```python
from build123d import *

# Parameters (mm, degrees)
SKETCH_1_W          = 45
SKETCH_1_H          = 40
EXTRUDE_1_DEPTH     = 20
SKETCH_2_W          = 45
SKETCH_2_H          = 10
CUT_EXTRUDE_1_DEPTH = 32
SKETCH_3_W          = 45
SKETCH_3_H          = 5
EXTRUDE_2_DEPTH     = 5
SKETCH_4_R          = 1.5
CUT_EXTRUDE_2_DEPTH = 44.934610502
CHAMFER_1_SIZE      = 10


with BuildPart() as part:
    # 草图1 → 凸台-拉伸1 (new body)
    with BuildSketch(Plane(origin=(0, 0, 0), x_dir=(1, 0, 0), z_dir=(0, 1, 0))):
        Rectangle(SKETCH_1_W, SKETCH_1_H)
    extrude(amount=EXTRUDE_1_DEPTH)

    # 草图2 → 切除-拉伸1 (cut)
    with BuildSketch(Plane(origin=(0, 0, -20), x_dir=(-1, 0, 0), z_dir=(0, 0, -1))):
        with Locations((0, 15)):
            Rectangle(SKETCH_2_W, SKETCH_2_H)
    extrude(amount=-CUT_EXTRUDE_1_DEPTH, mode=Mode.SUBTRACT)

    # 草图3 → 凸台-拉伸2 (add)
    with BuildSketch(Plane(origin=(0, 10, 0), x_dir=(1, 0, 0), z_dir=(0, 1, 0))):
        with Locations((0, 17.5)):
            Rectangle(SKETCH_3_W, SKETCH_3_H)
    extrude(amount=EXTRUDE_2_DEPTH)

    # 草图4 → 切除-拉伸2 (cut, through all)
    with BuildSketch(Plane(origin=(0, 0, 12), x_dir=(-1, 0, 0), z_dir=(0, 0, -1))):
        with Locations((0, 15)):
            Circle(SKETCH_4_R)
    extrude(amount=-CUT_EXTRUDE_2_DEPTH, mode=Mode.SUBTRACT)

    # 倒角1
    chamfer_1_edges = [part.edges().sort_by_distance(p)[0] for p in [
        (-22.5, 10, 20),
    ]]
    chamfer(chamfer_1_edges, length=CHAMFER_1_SIZE)


solid = part.part
```
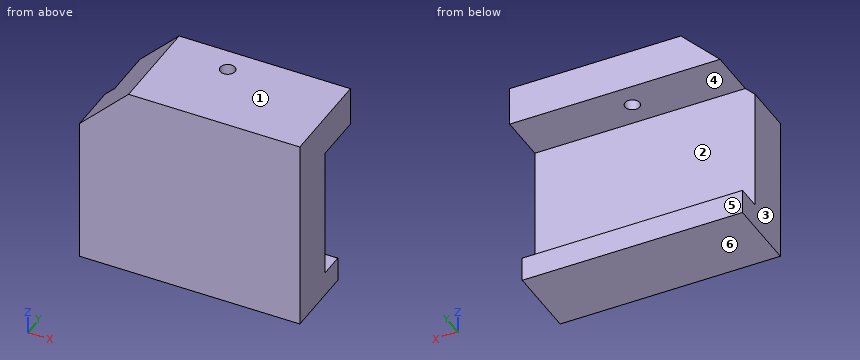
The model under review builds one solid part; all positions refer to its coordinate system, in mm. Face numbers are marked on the shaded views. A direction names the side the tool comes from. Give positions to 0.01 mm unless a question says otherwise; leave off trailing zeros. Loops run counter-clockwise (first coordinate to the right, second up) from the corner with the lowest first, then second, coordinate; pieces in that order, holes last. Notation, with made-up numbers: (11.25, 18) - (50.25, 18) arc R12 ccw to (50.25, 27) - close; hole circle Ø11 at (-5, 68.25). An arc over 180 degrees is marked (long way). Answer as a JSON object with one key per item and string values.
Q1. Add section A-A on x = 0. State the section outline as (y, z) points, plus the area to 3 significant figures.
Worked out:
{"outline": "(0, -20) - (15, -20) - (15, -15) - (10, -15) - (10, 12) - (13.5, 12) - (13.5, 20) - (0, 20) - close; (16.5, 12) - (20, 12) - (20, 20) - (16.5, 20) - close", "area": "481 mm^2"}
Q2. Mouldability with a two-part tool opening along Z and no side actions: class the marked faces 1, 2, 3 and 4 as +Z half, -Z half, draft (parallel to the pull), parting line (faces both ways), or undercut.
Worked out:
{"face 1": "+Z half", "face 2": "undercut", "face 3": "draft", "face 4": "undercut"}
Q3. Add section D-D on x = -8. State the section outline as (y, z) points.
Worked out:
{"outline": "(0, -20) - (15, -20) - (15, -15) - (10, -15) - (10, 12) - (20, 12) - (20, 20) - (0, 20) - close"}
Q4. To check wall thickness, follow line 1 along Y through (x, z) = (0, 16); line 2 along Z through (x, y) = (-10.5, 14); line 3 along Y through (x, z) = (7.5, 7.5). State the ranges of each line that lie inside material, in increasing order.
Worked out:
{"line 1": "y = 0 to 13.5, 16.5 to 20", "line 2": "z = -20 to -15, 12 to 20", "line 3": "y = 0 to 10"}
Q5. For the marked faces 5 and 6, list the 3-axis set-ups (+Z, -Z, +X, -X, +Y, -Y) from which the entire face can be reached by the end or side of a thin tool; tool diameter is ignored.
Worked out:
{"face 5": "-Z, +X, -X, +Y", "face 6": "-Z, +X, -X, +Y, -Y"}
Q6. Add section C-C on y = 11.75. State the section outline as (x, z) points.
Worked out:
{"outline": "(-22.5, -20) - (22.5, -20) - (22.5, -15) - (-22.5, -15) - close; (-20.5, 12) - (22.5, 12) - (22.5, 20) - (-12.5, 20) - close"}
Q7. Add section B-B on z = 14. State the section outline as (x, y) points.
Worked out:
{"outline": "(-18.5, 0) - (22.5, 0) - (22.5, 20) - (-18.5, 20) - close; hole circle Ø3 at (0, 15)"}
Q8. Insertion check: pin 1 (8 mm diameter, centred on x = -6.5, z = 4, fed in from +Y); pin 2 (4 mm diameter, centred on x = 3.5, z = -18.5, fed in from +Y). Each pin has a flat end and moves straight along its axis. Give the tip position at first contact, or say it passes through.
Worked out:
{"pin 1": "stops at y = 10", "pin 2": "stops at y = 15"}
